from build123d import *

# Parameters (mm, degrees)
BOSS_EXTRUDE1_DEPTH = 1.1
SKETCH3_W           = 11.9
SKETCH3_H           = 11
SKETCH3_W_2         = 5.4
SKETCH3_H_2         = 4
BOSS_EXTRUDE2_DEPTH = 1.1
SKETCH4_W           = 11.9
SKETCH4_H           = 11
SKETCH4_W_2         = 5.4
SKETCH4_H_2         = 4
BOSS_EXTRUDE3_DEPTH = 1.1
BOSS_EXTRUDE4_DEPTH = 4.25


with BuildPart() as part:
    # Sketch1 → Boss-Extrude1 (new body)
    with BuildSketch(Plane.XY):
        with BuildLine():
            Line((3.951985261, -6.654962537), (-3.971646211, -6.654962537))
            ThreePointArc((-3.971646211, -6.654962537), (-7.748260545, -0.1641905), (-4.25, 6.480740698))
            Line((-4.25, 6.480740698), (4.25, 6.468710372))
            ThreePointArc((4.25, 6.468710372), (7.737947933, -0.175714722), (3.951985261, -6.654962537))
        make_face()
        with BuildLine():
            Line((-3.388637081, -4.549455129), (3.388637081, -4.549455129))
            ThreePointArc((3.388637081, -4.549455129), (0, 5.672777383), (-3.388637081, -4.549455129))
        make_face(mode=Mode.SUBTRACT)
    extrude(amount=BOSS_EXTRUDE1_DEPTH)



with BuildPart() as body_2:
    # Sketch3 → Boss-Extrude2 (new body)
    with BuildSketch(Plane(origin=(0, -8.4, 0), x_dir=(-1, 0, 0), z_dir=(0, -1, 0))):
        with Locations((0, -17.45)):
            Rectangle(SKETCH3_W, SKETCH3_H)
        with Locations((0, -18.05)):
            Rectangle(SKETCH3_W_2, SKETCH3_H_2, mode=Mode.SUBTRACT)
    extrude(amount=BOSS_EXTRUDE2_DEPTH)


with BuildPart() as body_3:
    # Sketch4 → Boss-Extrude3 (new body)
    with BuildSketch(Plane(origin=(0, 8.5, 0), x_dir=(1, 0, 0), z_dir=(0, 1, 0))):
        with Locations((0, -17.45)):
            Rectangle(SKETCH4_W, SKETCH4_H)
        with Locations((0, -18.05)):
            Rectangle(SKETCH4_W_2, SKETCH4_H_2, mode=Mode.SUBTRACT)
    extrude(amount=BOSS_EXTRUDE3_DEPTH)


with BuildPart() as part_1:
    add(part.part)

    add(body_2.part)  # Boss-Extrude4 merges body 2

    add(body_3.part)  # Boss-Extrude4 merges body 3
    # Sketch2 → Boss-Extrude4 (add, symmetric)
    with BuildSketch(Plane(origin=(0, 0, 0), x_dir=(0, 0, -1), z_dir=(1, 0, 0))):
        with BuildLine():
            Line((-1.1, -6.245079779), (0, -6.245079779))
            Line((0, -6.245079779), (0, -8))
            ThreePointArc((0, -8), (-0.439339828, -9.060660172), (-1.5, -9.5))
            Line((-1.5, -9.5), (-11.95, -9.5))
            Line((-11.95, -9.5), (-11.95, -8.4))
            Line((-11.95, -8.4), (-2.6, -8.4))
            ThreePointArc((-2.6, -8.4), (-1.539339828, -7.960660172), (-1.1, -6.9))
            Line((-1.1, -6.9), (-1.1, -6.245079779))
        make_face()
        with BuildLine():
            Line((-1.1, 6.20982384), (0, 6.20982384))
            Line((0, 6.20982384), (0, 8.1))
            ThreePointArc((0, 8.1), (-0.439339828, 9.160660172), (-1.5, 9.6))
            Line((-1.5, 9.6), (-11.95, 9.6))
            Line((-11.95, 9.6), (-11.95, 8.5))
            Line((-11.95, 8.5), (-2.6, 8.5))
            ThreePointArc((-2.6, 8.5), (-1.539339828, 8.060660172), (-1.1, 7))
            Line((-1.1, 7), (-1.1, 6.20982384))
        make_face()
    extrude(amount=BOSS_EXTRUDE4_DEPTH, both=True)


solid = part_1.part
Geometry: final body of the model. Coordinates: model frame, mm. A direction names the side the tool comes from. Coordinates: 2 decimals unless noted, no trailing zeros. Loops run counter-clockwise (first coordinate to the right, second up) from the corner with the lowest first, then second, coordinate; pieces in that order, holes last. Notation, with made-up numbers: M -37,68.25 L -18,68.25 A31 cw -18,106.25 Z; hole C 84,-20.75 d10. An arc over 180 degrees is marked long. One line per item, written item: value. Start each with the question number.
1) Pin query (flat end, axial travel): P1, Ø3.5, axis at y = -7.5, z = 8, coming from the -X side; P2, Ø1.2, axis at y = 9.5, z = 17.5, coming from the +X side; P3, Ø3.5, axis at y = 7.5, z = 5, coming from the +X side. Return the tip coordinate at first contact, or that it passes through.
2) Cut plane D-D (y = -5.5). Return loops of the section in (x, z), then the cut area to 3 significant figures.
3) Draft query along X for faces 5 (the flat face through (-2.7, 9, 18)), 6 (the flat face through (-5.95, 9, 18)), 7 (the cylindrical face through (-0.06, -7.97, 1.55)). Return one class per face: released by +X, released by -X, zero draft, split by the parting line, or undercut.
4) Cut plane A-A (y = 0). Return loops of the section in (x, z).
5) Material intervals for L1, parallel to Y at x = -2.5, z = 13; L2, parallel to Z at x = -5.25, y = -4.25; L3, parallel to Y at x = 0, z = 0.3, sorted ascending. Write a range as from..to.
6) Reachability of faces 1 (the flat face through (4.25, 9, 5)), 2 (the flat face through (5, -9, 11.95)), 3 (the flat face through (0, -9, 20.05)), 4 (the flat face through (0, -8.4, 13)) from +Z, -Z, +X, -X, +Y, -Y: full face, straight path, thin tool, end or side. Return the list, or none.
7) Cut plane C-C (x = 0). Return loops of the section in (y, z).
8) Cut plane B-B (z = 7.75). Return loops of the section in (x, y), then the cut area to 3 significant figures.
Evaluation:
1. P1: x = -4.25
1. P2: x = 5.95
1. P3: x = 4.25
2. outline: M -5.46,0 L 5.45,0 L 5.45,1.1 L -5.46,1.1 Z
2. area: 12.0 mm^2
3. face 5: undercut
3. face 6: released by -X
3. face 7: zero draft
4. outline: M -7.75,0 L -5.67,0 L -5.67,1.1 L -7.75,1.1 Z; M 5.67,0 L 7.74,0 L 7.74,1.1 L 5.67,1.1 Z
5. L1: -9.5..-8.4, 8.5..9.6
5. L2: 0..1.1
5. L3: -8.9..-4.55, 5.67..9
6. face 1: -Z, +X, +Y
6. face 2: -Z, +X, +Y, -Y
6. face 3: +Y, -Y
6. face 4: +Z, +X, -X
7. outline: M -9.5,1.5 A1.5 ccw -8,0 L -4.55,0 L -4.55,1.1 L -6.9,1.1 A1.5 cw -8.4,2.6 L -8.4,16.05 L -9.5,16.05 Z; M -9.5,20.05 L -8.4,20.05 L -8.4,22.95 L -9.5,22.95 Z; M 5.67,0 L 8.1,0 A1.5 ccw 9.6,1.5 L 9.6,16.05 L 8.5,16.05 L 8.5,2.6 A1.5 cw 7,1.1 L 5.67,1.1 Z; M 8.5,20.05 L 9.6,20.05 L 9.6,22.95 L 8.5,22.95 Z
8. outline: M -4.25,-9.5 L 4.25,-9.5 L 4.25,-8.4 L -4.25,-8.4 Z; M -4.25,8.5 L 4.25,8.5 L 4.25,9.6 L -4.25,9.6 Z
8. area: 18.7 mm^2
